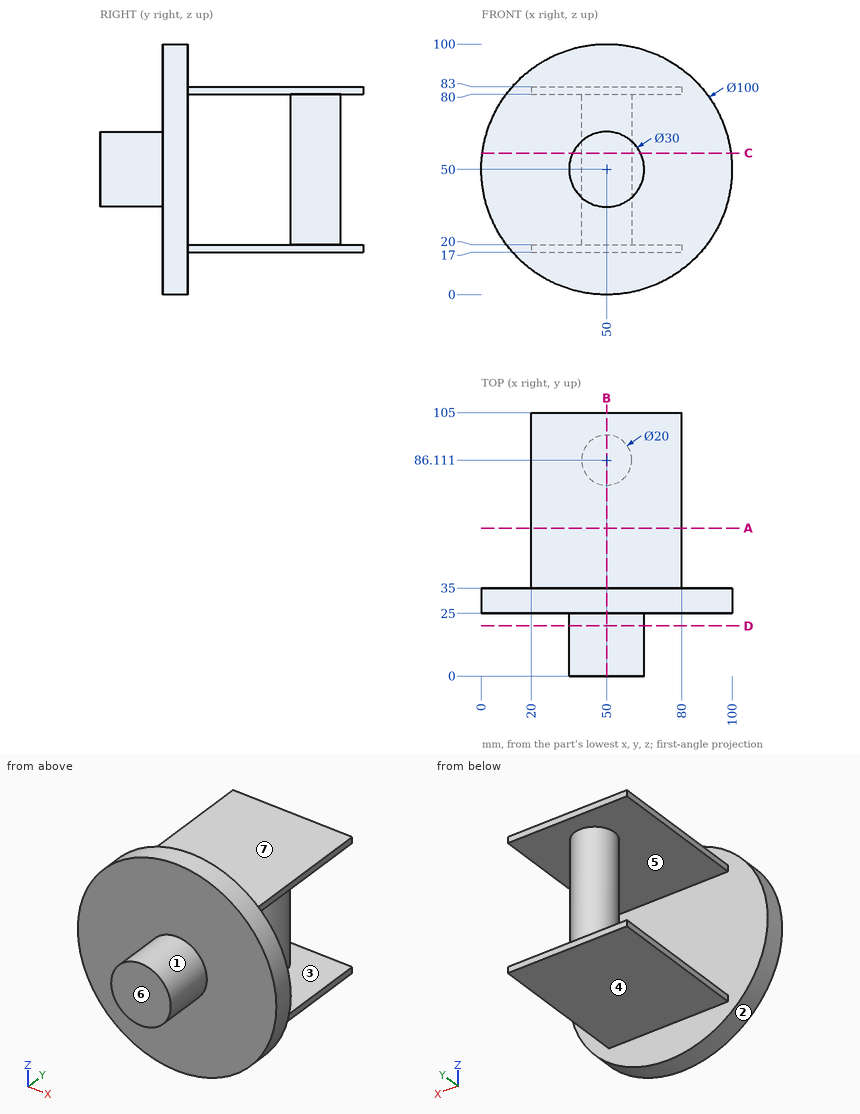
Check sheet for the drawn part. Datum: minimum x, y, z corner. Units: mm. A direction names the side the tool comes from. Give positions to 0.01 mm unless a question says otherwise; leave off trailing zeros. Order: outer loops, then holes, each group sorted by start corner. A loop starts at its lowest first (then second) coordinate and runs counter-clockwise, first axis right, second up. Notation, with made-up numbers: (85.25, 67.25) -> (91.25, 67.25) arc R19 cw to (91.25, 73.25) -> close; hole circle Ø3 at (32, 17). An arc over 180 degrees is marked (long way). Use a Markdown table: item, result.
1) Tool access check on the marked faces 1, 2, 3 and 4. Record the directions out of +Z, -Z, +X, -X, +Y, -Y that give a thin tool (end or side, any length) a straight path to the whole face; none if there is none.
Results:
| item | result |
|---|---|
| face 1 | -Y |
| face 2 | +Y, -Y |
| face 3 | none |
| face 4 | -Z, +X, -X, +Y |
2) Section check C-C, the plane z = 56.5. Record the boundary of the cut face in (x, y).
Results:
| item | result |
|---|---|
| outline | (0.42, 25) -> (36.48, 25) -> (36.48, 0) -> (63.52, 0) -> (63.52, 25) -> (99.58, 25) -> (99.58, 35) -> (0.42, 35) -> close; circle Ø20 at (50, 86.11) |
3) Section check B-B, the plane x = 50. Record the boundary of the cut face in (y, z).
Results:
| item | result |
|---|---|
| outline | (0, 35) -> (25, 35) -> (25, 0) -> (35, 0) -> (35, 17) -> (105, 17) -> (105, 20) -> (96.11, 20) -> (96.11, 80) -> (105, 80) -> (105, 83) -> (35, 83) -> (35, 100) -> (25, 100) -> (25, 65) -> (0, 65) -> close; hole (35, 20) -> (76.11, 20) -> (76.11, 80) -> (35, 80) -> close |
4) Material ranges on probe 1 along Z at (x, y) = (23, 82.5); probe 2 along Y at (x, z) = (20, 65); probe 3 along Z at (x, y) = (49, 32), recorded low to high.
Results:
| item | result |
|---|---|
| probe 1 | 17 to 20, 80 to 83 |
| probe 2 | 25 to 35 |
| probe 3 | 0.01 to 99.99 |
5) Depth check by flat-ended pin: pin 1 Ø12 at (x, y) = (76.5, 91.5) entering from +Z; pin 2 Ø2.5 at (y, z) = (65, 18.5) entering from -X; pin 3 Ø3.5 at (y, z) = (86, 18.5) entering from +X. Enter the tip coordinate at first touch or a pass-through.
Results:
| item | result |
|---|---|
| pin 1 | z = 83 |
| pin 2 | x = 20 |
| pin 3 | x = 80 |
6) Section check A-A, the plane y = 59. Record the boundary of the cut face in (x, z), then the cut area to 3 significant figures.
Results:
| item | result |
|---|---|
| outline | (20, 17) -> (80, 17) -> (80, 20) -> (20, 20) -> close; (20, 80) -> (80, 80) -> (80, 83) -> (20, 83) -> close |
| area | 360 mm² |
7) Mould release check, pull along Z, two halves, no side actions. Record for the marked faces 5, 6 and 7: pulls with the +Z half, pulls with the -Z half, needs draft (parallel to the pull), parting line crosses it, or undercut.
Results:
| item | result |
|---|---|
| face 5 | undercut |
| face 6 | needs draft |
| face 7 | pulls with the +Z half |
8) Section check D-D, the plane y = 20. Record the boundary of the cut face in (x, z).
Results:
| item | result |
|---|---|
| outline | circle Ø30 at (50, 50) |
